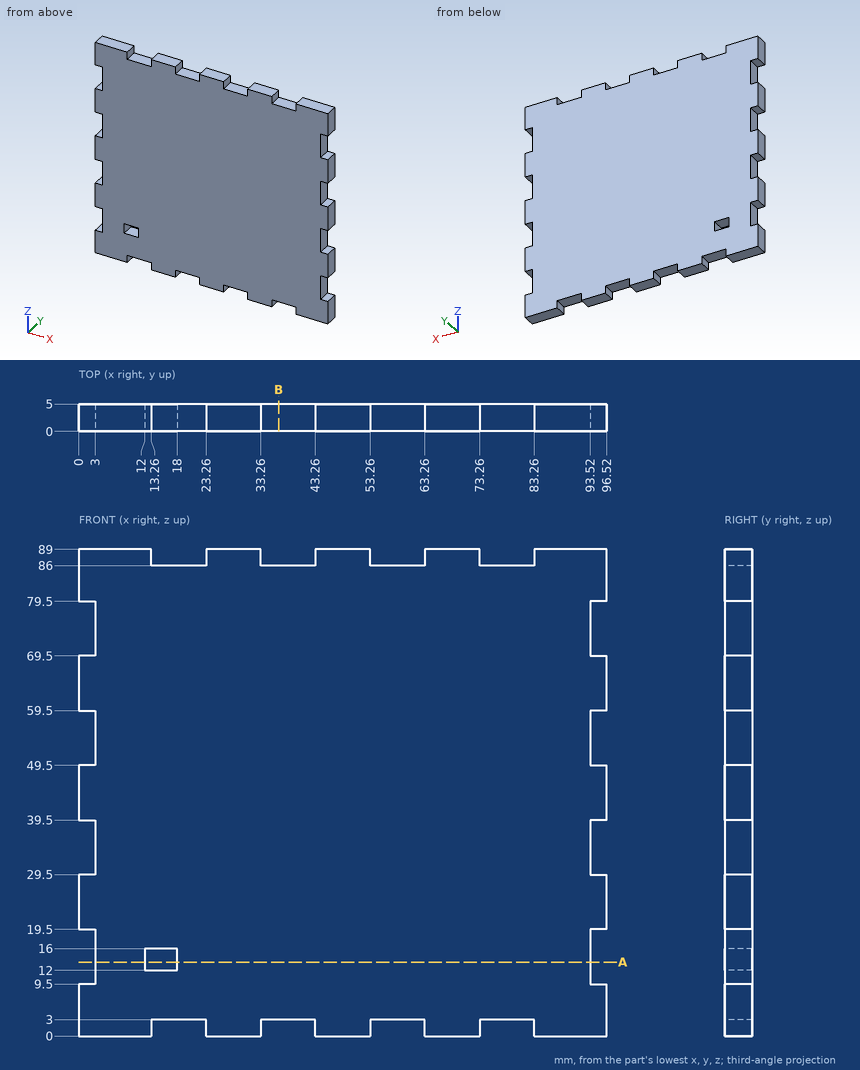
Can you work these out from the drawing? Everything is in mm from the part's minimum corner. Coordinates: 2 decimals unless noted, no trailing zeros. Loops run counter-clockwise (first coordinate to the right, second up) from the corner with the lowest first, then second, coordinate; pieces in that order, holes last.
1) Imagine slicing it at A-A (z = 13.5). List the corners of the cut face in (x, y) for me, and give its area (3 significant figures).
Reported:
outline: (3, 0) - (12, 0) - (12, 5) - (3, 5) - close; (18, 0) - (93.52, 0) - (93.52, 5) - (18, 5) - close
area: 423 mm2
2) Please list where these lines run through material, in increasing order: line 1 along X through (y, z) = (0.75, 12.5); line 2 along X through (y, z) = (1.8, 50.5); line 3 along Z through (x, y) = (34.5, 0.6).
Reported:
line 1: x = 3 to 12, 18 to 93.52
line 2: x = 3 to 93.52
line 3: z = 3 to 86
3) Imagine slicing it at B-B (x = 36.5). List the corners of the cut face in (y, z) for me, and give its area (3 significant figures).
Reported:
outline: (0, 3) - (5, 3) - (5, 86) - (0, 86) - close
area: 415 mm2
4) Will this pin go through, and if not, where does the flat tip stop? pin 1 Ø2.5 at (x, y) = (37.5, 2.5) entering from +Z.
Reported:
pin 1: stops at z = 86
